Verification items for the finished model (mm, model axes). Give positions to 0.01 mm unless a question says otherwise; leave off trailing zeros. Write each loop counter-clockwise with the first axis right and the second up, starting at its lowest first coordinate (ties: lowest second). Pieces come first, ordered by that corner, then holes. Notation, with made-up numbers: (38.25, 24.5) -> (49.25, 24.5) arc R26 cw to (49.25, 44.5) -> close; hole circle Ø8 at (9.25, -1). An arc over 180 degrees is marked (long way). Use one line per item in the form item = value. Start each with the question number.
(1) Scan lines: L1, parallel to Y at x = 1, z = 3096.5; L2, parallel to Z at x = -11.5, y = -17.5. Record each from-to range of solid material in increasing order.
(2) Section check A-A, the plane z = 3110. Record the cut outline in (x, y), plus the area to 4 significant figures.
(3) Depth check by flat-ended pin: pin 1 Ø2 at (x, y) = (-21.5, -72.5) entering from -Z; pin 2 Ø17.5 at (y, z) = (-69, 3311) entering from +X; pin 3 Ø13.5 at (y, z) = (8.5, 1496) entering from -X. Enter the tip coordinate at first touch or a pass-through.
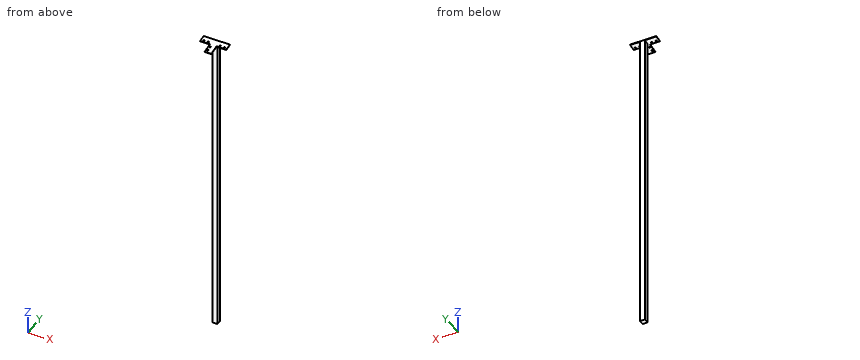
from build123d import *

# Parameters (mm, degrees)
F0_W      = 45
F0_H      = 45
F1_DEPTH  = 3330
F6_W      = 45
F6_H      = 45.842251273
F7_DEPTH  = 25
F8_W      = 60
F8_H      = 60
F8_W_2    = 90
F8_H_2    = 90
F9_DEPTH  = 5
F10_R     = 6
F11_DEPTH = 25
F12_W     = 150
F12_H     = 4.7702248844
F13_DEPTH = 3358.6871623993
F15_DEPTH = 106.2
F16_W     = 45
F16_H     = 45
F17_DEPTH = 534


with BuildPart() as f1:
    # F0 (on Top) → F1 (new body)
    with BuildSketch(Plane.XY):
        Rectangle(F0_W, F0_H)
    extrude(amount=F1_DEPTH)

    # F6 (on face) → F7 (join)
    with BuildSketch(Plane(origin=(0, -624.5391596736, 3212.9754420296), x_dir=(1, 0, 0), z_dir=(0, 0.1908089954, -0.9816271834))):
        with Locations((0, -636.2284686128)):
            Rectangle(F6_W, F6_H)
    extrude(amount=F7_DEPTH)

    # F8 (on face) → F9 (join)
    with BuildSketch(Plane(origin=(0, -624.5391596736, 3212.9754420296), x_dir=(1, 0, 0), z_dir=(0, 0.1908089954, -0.9816271834))):
        with Locations((-7.5, -629.1495942493)):
            Rectangle(F8_W, F8_H)
        with Locations((-82.5, -629.1495942493)):
            Rectangle(F8_W_2, F8_H)
        with Locations((67.5, -629.1495942493)):
            Rectangle(F8_W_2, F8_H)
        with Locations((-7.5, -554.1495942493)):
            Rectangle(F8_W, F8_H_2)
    extrude(amount=F9_DEPTH)

    # F10 (on face) → F11 (cut)
    with BuildSketch(Plane(origin=(0, -624.5391596736, 3212.9754420296), x_dir=(1, 0, 0), z_dir=(0, -0.1908089954, 0.9816271834))):
        with BuildLine():
            ThreePointArc((81.5, 614.1495942493), (83.2573593129, 609.9069535622), (87.5, 608.1495942493))
            Line((87.5, 608.1495942493), (87.5, 614.1495942493))
            Line((87.5, 614.1495942493), (81.5, 614.1495942493))
        make_face()
        with Locations((47.5, 614.1495942493)):
            Circle(F10_R)
        with BuildLine():
            Line((87.5, 614.1495942493), (87.5, 608.1495942493))
            ThreePointArc((87.5, 608.1495942493), (91.7426406871, 609.9069535622), (93.5, 614.1495942493))
            ThreePointArc((93.5, 614.1495942493), (87.5, 620.1495942493), (81.5, 614.1495942493))
            Line((81.5, 614.1495942493), (87.5, 614.1495942493))
        make_face()
        with BuildLine():
            ThreePointArc((-22.5, 540.1495942493), (-28.5, 534.1495942493), (-22.5, 528.1495942493))
            Line((-22.5, 528.1495942493), (-22.5, 540.1495942493))
        make_face()
        with BuildLine():
            ThreePointArc((-22.5, 580.1495942493), (-28.5, 574.1495942493), (-22.5, 568.1495942493))
            Line((-22.5, 568.1495942493), (-22.5, 580.1495942493))
        make_face()
        with BuildLine():
            Line((-22.5, 580.1495942493), (-22.5, 568.1495942493))
            ThreePointArc((-22.5, 568.1495942493), (-18.2573593129, 569.9069535622), (-16.5, 574.1495942493))
            ThreePointArc((-16.5, 574.1495942493), (-18.2573593129, 578.3922349364), (-22.5, 580.1495942493))
        make_face()
        with BuildLine():
            Line((-22.5, 540.1495942493), (-22.5, 528.1495942493))
            ThreePointArc((-22.5, 528.1495942493), (-18.2573593129, 529.9069535622), (-16.5, 534.1495942493))
            ThreePointArc((-16.5, 534.1495942493), (-18.2573593129, 538.3922349364), (-22.5, 540.1495942493))
        make_face()
        with Locations((-62.5, 614.1495942493)):
            Circle(F10_R)
        with Locations((-102.5, 614.1495942493)):
            Circle(F10_R)
    extrude(amount=-F11_DEPTH, mode=Mode.SUBTRACT)

    # F12 (on Top) → F13 (cut)
    with BuildSketch(Plane.XY):
        with Locations((52.5, 24.8851124422)):
            Rectangle(F12_W, F12_H)
    extrude(amount=F13_DEPTH, mode=Mode.SUBTRACT)

    # F14 (on face) → F15 (cut)
    with BuildSketch(Plane.YZ.offset(-22.5)):
        Polygon((22.5, 3338.7471139112), (22.5, 3333.6535304364), (23.4540449769, 3333.838977994), align=None)
    extrude(amount=-F15_DEPTH, mode=Mode.SUBTRACT)

    # F16 (on face) → F17 (cut)
    with BuildSketch(Plane(origin=(0, 0, 0), x_dir=(1, 0, 0), z_dir=(0, 0, -1))):
        Rectangle(F16_W, F16_H)
    extrude(amount=-F17_DEPTH, mode=Mode.SUBTRACT)


solid = f1.part
Completed:
q1.L1 = -22.5 to 22.5
q1.L2 = 534 to 3330.97
q2.outline = (-22.5, -22.5) -> (22.5, -22.5) -> (22.5, 22.5) -> (-22.5, 22.5) -> close
q2.area = 2,025 mm²
q3.pin_1 = 3314.99
q3.pin_2 = 22.5
q3.pin_3 = -22.5
